Geometry: final body of the model. Coordinates: model frame, mm. Give positions to 0.01 mm unless a question says otherwise; leave off trailing zeros. One line per question, with ' | ' between items. Start each with the question number.
(1) Mould query, pull axis X, two halves, no side actions, for faces 1 (the face through (325, 246, 0)), 2 (the face through (164.938, 101.954, 7.465)). Classes: +X half, -X half, draft (parallel to the pull), parting line (faces both ways), or undercut.
(2) Ray query, L1, parallel to X at y = 181, z = 7.5; L2, parallel to Y at x = 230.5, z = 8.75; L3, parallel to Y at x = 274, z = 9.75. Return the intervals inside material, ascending.
(3) First-contact query: pin 1 Ø12 at (x, y) = (115, 366.5) entering from +Z. Flat tip, straight axial feed; report the tip coordinate or a pass-through.
```python
from build123d import *

# Parameters (mm, degrees)
ESQUISSE1_W             = 660
ESQUISSE1_H             = 485
BOSS_EXTRU_1_DEPTH      = 10
ENL_V_MAT_EXTRU_1_DEPTH = 5
CHANFREIN1_SIZE         = 5


with BuildPart() as part:
    # Esquisse1 → Boss.-Extru.1 (new body)
    with BuildSketch(Plane.XY):
        with Locations((330, 242.5)):
            Rectangle(ESQUISSE1_W, ESQUISSE1_H)
    extrude(amount=BOSS_EXTRU_1_DEPTH)

    # Esquisse2 → Enlèv. mat.-Extru.1 (cut)
    with BuildSketch(Plane.XY.offset(10)):
        Polygon((120, 208.994949366), (120, 276.005050634), (60, 336.005050634), (60, 148.994949366), align=None)
        Polygon((218.994949366, 375), (441.005050634, 375), (491.005050634, 425), (168.994949366, 425), align=None)
        Polygon((60, 425), (60, 378.431457505), (150, 288.431457505), (150, 196.568542495), (60, 106.568542495), (60, 60), (126.568542495, 60), (206.568542495, 140), (453.431457505, 140), (533.431457505, 60), (600, 60), (600, 106.568542495), (510, 196.568542495), (510, 288.431457505), (600, 378.431457505), (600, 425), (533.431457505, 425), (453.431457505, 345), (206.568542495, 345), (126.568542495, 425), align=None)
        Polygon((540, 208.994949366), (540, 276.005050634), (600, 336.005050634), (600, 148.994949366), align=None)
        Polygon((491.005050634, 60), (168.994949366, 60), (218.994949366, 110), (441.005050634, 110), align=None)
    extrude(amount=-ENL_V_MAT_EXTRU_1_DEPTH, mode=Mode.SUBTRACT)

    # Chanfrein1
    chanfrein1_edges = [part.edges().sort_by_distance(p)[0] for p in [
        (330, 60, 5),
        (193.994949366, 85, 5),
        (330, 110, 5),
        (466.005050634, 85, 5),
        (60, 242.5, 5),
        (90, 306.005050634, 5),
        (120, 242.5, 5),
        (90, 178.994949366, 5),
        (600, 242.5, 5),
        (570, 178.994949366, 5),
        (540, 242.5, 5),
        (570, 306.005050634, 5),
        (166.568542495, 385, 5),
        (330, 345, 5),
        (493.431457505, 385, 5),
        (566.715728753, 425, 5),
        (600, 401.715728753, 5),
        (555, 333.431457505, 5),
        (510, 242.5, 5),
        (555, 151.568542495, 5),
        (600, 83.284271247, 5),
        (566.715728753, 60, 5),
        (493.431457505, 100, 5),
        (330, 140, 5),
        (166.568542495, 100, 5),
        (93.284271247, 60, 5),
        (60, 83.284271247, 5),
        (105, 151.568542495, 5),
        (150, 242.5, 5),
        (105, 333.431457505, 5),
        (60, 401.715728753, 5),
        (93.284271247, 425, 5),
        (330, 425, 5),
        (466.005050634, 400, 5),
        (330, 375, 5),
        (193.994949366, 400, 5),
    ]]
    chamfer(chanfrein1_edges, length=CHANFREIN1_SIZE - 0.0001)  # a hair under: the kernel refuses the full size


solid = part.part
```
Response:
1) face 1: draft | face 2: undercut
2) L1: x = 0 to 62.5, 88.47 to 137.97, 522.03 to 571.53, 597.5 to 660 | L2: y = 0 to 61.25, 108.75 to 141.25, 343.75 to 376.25, 423.75 to 485 | L3: y = 0 to 60.25, 109.75 to 140.25, 344.75 to 375.25, 424.75 to 485
3) pin 1: stops at z = 5
